from build123d import *

# Parameters (mm, degrees)
F0_W          = 25
F0_H          = 15
F2_R          = 23.4773699194
F3_DEPTH      = 18.22955
F4_W          = 30
F4_H          = 20
F5_DEPTH      = 30
F5_DEPTH_BACK = 30
F7_R          = 1.3613777444
F9_W          = 3
F9_H          = 3
F10_DEPTH     = 60


with BuildPart() as f1:
    # F0 (on Front) → F1 (revolve)
    with BuildSketch(Plane.XZ):
        with Locations((-12.5, 7.5)):
            Rectangle(F0_W, F0_H)
    revolve(axis=Axis((0, 0, 7.5), (0, 0, 1)))

    # F2 (on face) → F3 (cut)
    with BuildSketch(Plane.XY.offset(15)):
        Circle(F2_R)
    extrude(amount=-F3_DEPTH, mode=Mode.SUBTRACT)

    # F4 (on Front) → F5 (join, two sides)
    with BuildSketch(Plane.XZ) as f5_sk:
        with Locations((15, -10)):
            Rectangle(F4_W, F4_H)
        with Locations((-15, -10)):
            Rectangle(F4_W, F4_H)
    extrude(amount=F5_DEPTH)
    extrude(f5_sk.sketch, amount=-F5_DEPTH_BACK)

    # F8: sweep along a path in F6
    with BuildLine(Plane.XZ) as f8_path:
        Line((27.4984519929, 0), (27.4984519929, 32))
        ThreePointArc((27.4984519929, 32), (26.9126655552, 33.4142135624), (25.4984519929, 34))
        Line((25.4984519929, 34), (10.4984519929, 34))
    # F7 (on Top) → F8 (sweep)
    with BuildSketch(Plane.XY):
        with Locations((27.4991728365, 0)):
            Circle(F7_R)
    sweep(path=f8_path.line)

    # F9 (on face) → F10 (join)
    with BuildSketch(Plane(origin=(0, 0, -20), x_dir=(1, 0, 0), z_dir=(0, 0, -1))):
        with Locations((-28.5, 28.5)):
            Rectangle(F9_W, F9_H)
        with Locations((28.5, 28.5)):
            Rectangle(F9_W, F9_H)
        with Locations((-28.5, -28.5)):
            Rectangle(F9_W, F9_H)
        with Locations((28.5, -28.5)):
            Rectangle(F9_W, F9_H)
    extrude(amount=F10_DEPTH)


solid = f1.part
Input: part model. Units: mm. Frame: model coordinates. A direction names the side the tool comes from. Round coordinates to 2 decimals unless told otherwise and drop trailing zeros. Order: outer loops, then holes, each group sorted by start corner. A loop starts at its lowest first (then second) coordinate and runs counter-clockwise, first axis right, second up. Notation, with made-up numbers: (5.5, -31.75) - (55.5, -31.75) arc R32 ccw to (55.5, 0.25) - close; hole circle Ø7 at (-14, 26). An arc over 180 degrees is marked (long way). Answer as a JSON object with one key per item and string values. Group by question number.
(1) Material intervals for probe 1 along Y at (x, z) = (0, 8); probe 2 along Z at (x, y) = (6.5, -7); probe 3 along X at (y, z) = (-20.5, 3), sorted ascending. Write a range as from..to.
(2) Cut plane B-B (y = 0). Return loops of the section in (x, z), then the cut area to 3 significant figures.
(3) Cut plane C-C (z = 6.5). Return loops of the section in (x, y).
(4) Pin query (flat end, axial travel): P1, Ø15, axis at x = -9.5, y = -10, coming from the +Z side; P2, Ø4, axis at x = -20.5, z = 1, coming from the +Y side; P3, Ø2, axis at y = -0.5, z = 34.5, coming from the -X side; P4, Ø12, axis at y = 22.5, z = 13, coming from the +X side. Return the tip coordinate at first contact, or that it passes through.
(5) Reachability of faces 1 (the face through (10.498, 0, 34)), 2 (the face through (28, 27, -50)), 3 (the face through (-29, 28, -80)), 4 (the face through (-27, -28, -50)), 5 (the face through (17.89, -0.52, 35.26)) from +Z, -Z, +X, -X, +Y, -Y: full face, straight path, thin tool, end or side. Return the list, or none.
(6) Cut plane D-D (x = 21). Return loops of the section in (y, z), then the cut area to 3 significant figures.
(7) Cut plane A-A (x = 0). Return loops of the section in (y, z).
(8) Draft query along Y for faces 6 (the face through (-30, 0, -16)), 7 (the face through (-29, 27, -50)), 8 (the face through (0, 30, -16)), 9 (the face through (-29, -27, -50)). Return one class per face: released by +Y, released by -Y, zero draft, split by the parting line, or undercut.
Here are the results:
{
 "1": {"probe 1": "y = -25..-23.48, 23.48..25", "probe 2": "z = -20..0", "probe 3": "x = -14.31..-11.44, 11.44..14.31"},
 "2": {"outline": "(-30, -20) - (30, -20) - (30, 0) - (28.86, 0) - (28.86, 32) arc R3.36 ccw to (25.5, 35.36) - (10.5, 35.36) - (10.5, 32.64) - (25.5, 32.64) arc R0.64 cw to (26.14, 32) - (26.14, 0) - (25, 0) - (25, 15) - (23.48, 15) - (23.48, 0) - (-23.48, 0) - (-23.48, 15) - (-25, 15) - (-25, 0) - (-30, 0) - close", "area": "1,380 mm^2"},
 "3": {"outline": "circle Ø50 at (0, 0); circle Ø2.72 at (27.5, 0); hole circle Ø46.95 at (0, 0)"},
 "4": {"P1": "stops at z = 0", "P2": "stops at y = 30", "P3": "stops at x = 10.5", "P4": "stops at x = 18.78"},
 "5": {"face 1": "+Z, -X, +Y, -Y", "face 2": "-Z, +X, -X", "face 3": "-Z, +X, -X, +Y, -Y", "face 4": "-Z, +Y, -Y", "face 5": "-X"},
 "6": {"outline": "(-30, -20) - (30, -20) - (30, 0) - (13.56, 0) - (13.56, 15) - (10.5, 15) - (10.5, 0) - (-10.5, 0) - (-10.5, 15) - (-13.56, 15) - (-13.56, 0) - (-30, 0) - close; circle Ø2.72 at (0, 34)", "area": "1,300 mm^2"},
 "7": {"outline": "(-30, -20) - (30, -20) - (30, 0) - (25, 0) - (25, 15) - (23.48, 15) - (23.48, 0) - (-23.48, 0) - (-23.48, 15) - (-25, 15) - (-25, 0) - (-30, 0) - close"},
 "8": {"face 6": "zero draft", "face 7": "undercut", "face 8": "released by +Y", "face 9": "undercut"}
}
